Input: dimensioned drawing with shaded views. Units: mm. Origin: part minimum x, y, z. Give positions to 0.01 mm unless a question says otherwise; leave off trailing zeros. Order: outer loops, then holes, each group sorted by start corner. A loop starts at its lowest first (then second) coordinate and runs counter-clockwise, first axis right, second up. Notation, with made-up numbers: (70.5, 3) - (81.5, 3) arc R14 ccw to (81.5, 29) - close; hole circle Ø2 at (-24, 81.25). An arc over 180 degrees is marked (long way). Use a Markdown table: item, result.
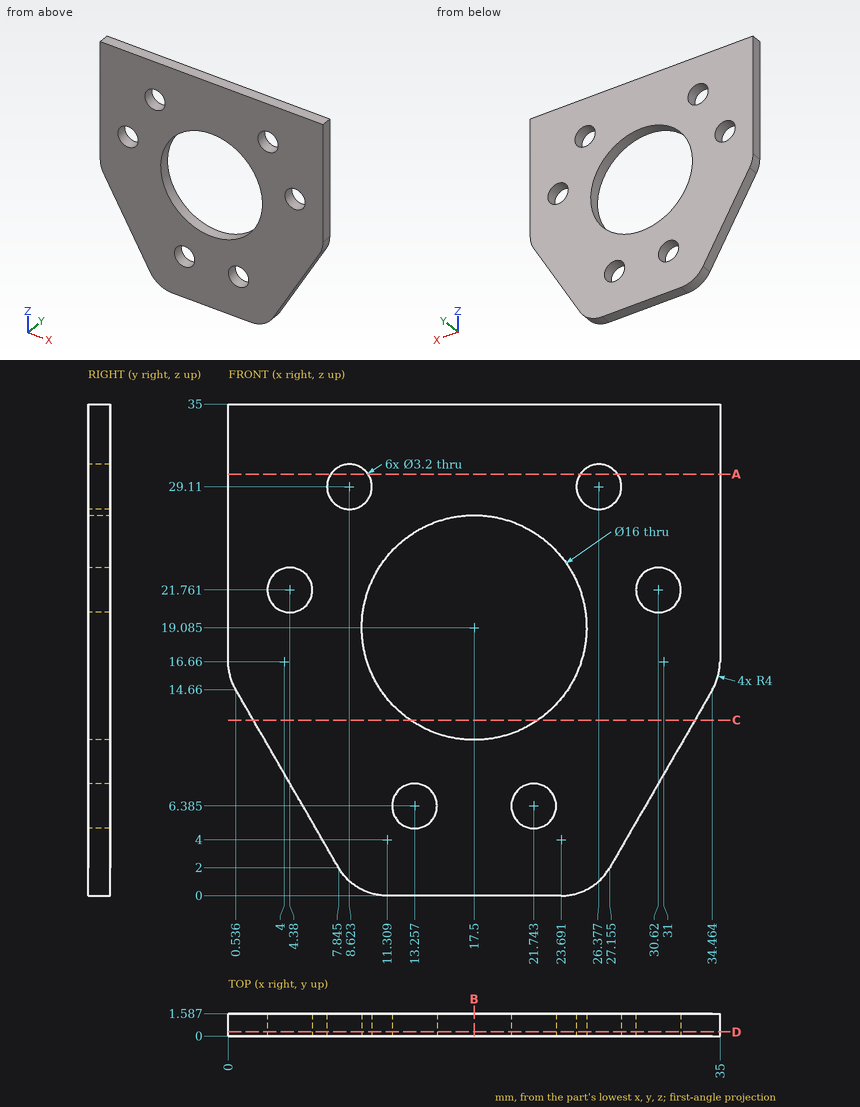
1. Section query D-D (y = 0.3). Return loops of the section in (x, z) (1 decimal).
Response:
| item | result |
|---|---|
| outline | (0, 16.7) arc R4 ccw to (0.5, 14.7) - (7.8, 2) arc R4 ccw to (11.3, 0) - (23.7, 0) arc R4 ccw to (27.2, 2) - (34.5, 14.7) arc R4 ccw to (35, 16.7) - (35, 35) - (0, 35) - close; hole circle Ø3.2 at (4.4, 21.8); hole circle Ø3.2 at (8.6, 29.1); hole circle Ø16 at (17.5, 19.1); hole circle Ø3.2 at (13.3, 6.4); hole circle Ø3.2 at (21.7, 6.4); hole circle Ø3.2 at (26.4, 29.1); hole circle Ø3.2 at (30.6, 21.8) |
2. Pin query (flat end, axial travel): pin 1 (2.5 mm diameter, centred on x = 8.62, z = 29.11, fed in from -Y). Return the tip coordinate at first contact, or that it passes through.
Response:
| item | result |
|---|---|
| pin 1 | passes through |
3. Section query C-C (z = 12.5). Return loops of the section in (x, y).
Response:
| item | result |
|---|---|
| outline | (1.78, 0) - (12.96, 0) - (12.96, 1.59) - (1.78, 1.59) - close; (22.04, 0) - (33.22, 0) - (33.22, 1.59) - (22.04, 1.59) - close |
4. Section query A-A (z = 30). Return loops of the section in (x, y).
Response:
| item | result |
|---|---|
| outline | (0, 0) - (7.29, 0) - (7.29, 1.59) - (0, 1.59) - close; (9.95, 0) - (25.05, 0) - (25.05, 1.59) - (9.95, 1.59) - close; (27.71, 0) - (35, 0) - (35, 1.59) - (27.71, 1.59) - close |
5. Material intervals for line 1 along Z through (x, y) = (13, 0.9) (1 decimal); line 2 along Z through (x, y) = (21.5, 0.9) (1 decimal); line 3 along X through (y, z) = (0.75, 20.5) (1 decimal), sorted ascending.
Response:
| item | result |
|---|---|
| line 1 | z = 0 to 4.8, 8 to 12.5, 25.7 to 35 |
| line 2 | z = 0 to 4.8, 8 to 12.2, 26 to 35 |
| line 3 | x = 0 to 3.4, 5.4 to 9.6, 25.4 to 29.6, 31.6 to 35 |
6. Section query B-B (x = 17.5). Return loops of the section in (y, z) (1 decimal).
Response:
| item | result |
|---|---|
| outline | (0, 0) - (1.6, 0) - (1.6, 11.1) - (0, 11.1) - close; (0, 27.1) - (1.6, 27.1) - (1.6, 35) - (0, 35) - close |
